Model file for the job. Use its own axes, mm. Face numbers are marked on the shaded views. Give positions to 0.01 mm unless a question says otherwise; leave off trailing zeros. Order: outer loops, then holes, each group sorted by start corner. A loop starts at its lowest first (then second) coordinate and runs counter-clockwise, first axis right, second up. Notation, with made-up numbers: (-24.75, -39) -> (30.25, -39) arc R24 ccw to (30.25, -29) -> close; hole circle Ø2 at (15.5, -36.75). An arc over 180 degrees is marked (long way). Answer in a Markdown table with one row per item. Add a question column.
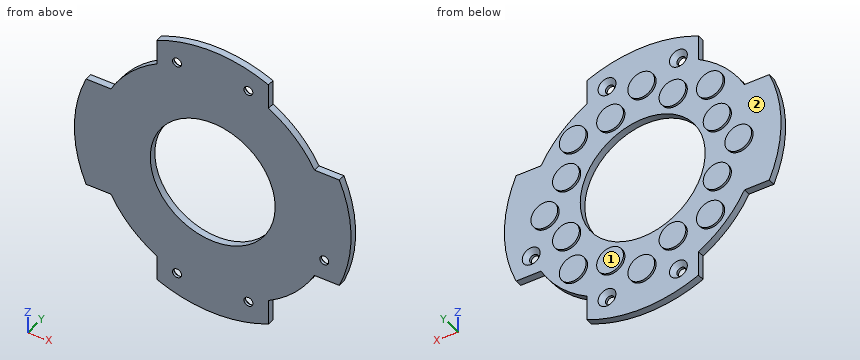
from build123d import *

# Parameters (mm, degrees)
SKETCH1_R           = 7
BOSS_EXTRUDE1_DEPTH = 0.7874
SKETCH2_R           = 1.5
BOSS_EXTRUDE2_DEPTH = 0.25
SKETCH3_R           = 0.5
CUT_EXTRUDE1_DEPTH  = 1.7874
CHAMFER1_SIZE       = 0.5


with BuildPart() as part:
    # Sketch1 → Boss-Extrude1 (new body)
    with BuildSketch(Plane(origin=(0, 0, 0), x_dir=(1, 0, 0), z_dir=(0, 1, 0))):
        with BuildLine():
            Line((-6.25, 14.184057953), (-6.25, 11.399013115))
            ThreePointArc((-6.25, 11.399013115), (-9.192388155, 9.192388155), (-11.399013115, 6.25))
            Line((-11.399013115, 6.25), (-14.184057953, 6.25))
            ThreePointArc((-14.184057953, 6.25), (-15.5, 0), (-14.184057953, -6.25))
            Line((-14.184057953, -6.25), (-11.399013115, -6.25))
            ThreePointArc((-11.399013115, -6.25), (-9.192388155, -9.192388155), (-6.25, -11.399013115))
            Line((-6.25, -11.399013115), (-6.25, -14.184057953))
            ThreePointArc((-6.25, -14.184057953), (0, -15.5), (6.25, -14.184057953))
            Line((6.25, -14.184057953), (6.25, -11.399013115))
            ThreePointArc((6.25, -11.399013115), (9.192388155, -9.192388155), (11.399013115, -6.25))
            Line((11.399013115, -6.25), (14.184057953, -6.25))
            ThreePointArc((14.184057953, -6.25), (15.5, 0), (14.184057953, 6.25))
            Line((14.184057953, 6.25), (11.399013115, 6.25))
            ThreePointArc((11.399013115, 6.25), (9.192388155, 9.192388155), (6.25, 11.399013115))
            Line((6.25, 11.399013115), (6.25, 14.184057953))
            ThreePointArc((6.25, 14.184057953), (0, 15.5), (-6.25, 14.184057953))
        make_face()
        Circle(SKETCH1_R, mode=Mode.SUBTRACT)
    extrude(amount=BOSS_EXTRUDE1_DEPTH)

    # Sketch2 → Boss-Extrude2 (add)
    with BuildSketch(Plane(origin=(0, 0.7874, 0), x_dir=(1, 0, 0), z_dir=(0, 1, 0))):
        with Locations((0, 10.865)):
            Circle(SKETCH2_R)
        with Locations((-3.495813155, 8.439639529)):
            Circle(SKETCH2_R)
        with Locations((-10.865, 0)):
            Circle(SKETCH2_R)
        with Locations((-8.439639529, 3.495813155)):
            Circle(SKETCH2_R)
        with Locations((-7.682715178, 7.682715178)):
            Circle(SKETCH2_R)
        with Locations((0, -10.865)):
            Circle(SKETCH2_R)
        with Locations((-3.495813155, -8.439639529)):
            Circle(SKETCH2_R)
        with Locations((-7.682715178, -7.682715178)):
            Circle(SKETCH2_R)
        with Locations((-8.439639529, -3.495813155)):
            Circle(SKETCH2_R)
        with Locations((3.495813155, 8.439639529)):
            Circle(SKETCH2_R)
        with Locations((7.682715178, 7.682715178)):
            Circle(SKETCH2_R)
        with Locations((8.439639529, 3.495813155)):
            Circle(SKETCH2_R)
        with Locations((10.865, 0)):
            Circle(SKETCH2_R)
        with Locations((8.439639529, -3.495813155)):
            Circle(SKETCH2_R)
        with Locations((7.682715178, -7.682715178)):
            Circle(SKETCH2_R)
        with Locations((3.495813155, -8.439639529)):
            Circle(SKETCH2_R)
    extrude(amount=BOSS_EXTRUDE2_DEPTH)

    # Sketch3 → Cut-Extrude1 (cut, through all)
    with BuildSketch(Plane(origin=(0, 0.7874, 0), x_dir=(1, 0, 0), z_dir=(0, 1, 0))):
        with Locations((-4, 12.5)):
            Circle(SKETCH3_R)
        with Locations((4, 12.5)):
            Circle(SKETCH3_R)
        with Locations((4, -12.5)):
            Circle(SKETCH3_R)
        with Locations((-4, -12.5)):
            Circle(SKETCH3_R)
        with Locations((12.5, 4)):
            Circle(SKETCH3_R)
    extrude(amount=-CUT_EXTRUDE1_DEPTH, mode=Mode.SUBTRACT)

    # Chamfer1
    chamfer1_edges = [part.edges().sort_by_distance(p)[0] for p in [
        (-4.5, 0.7874, -12.5),
        (3.5, 0.7874, -12.5),
        (3.5, 0.7874, 12.5),
        (-4.5, 0.7874, 12.5),
        (12, 0.7874, -4),
    ]]
    chamfer(chamfer1_edges, length=CHAMFER1_SIZE)


solid = part.part
Item 1: Two-plate mould, pull along X, no slides. Class the marked faces 1 and 2: pulls with the +X half, pulls with the -X half, needs draft (parallel to the pull), parting line crosses it, or undercut.
Item 2: Saw through at B-B on x = 0. List the corners of the cut face in (y, z) (3 decimals), plus the area to 3 significant figures.
Item 3: Saw through at A-A on z = 0. List the corners of the cut face in (x, y) (3 decimals), plus the area to 3 significant figures.
Item 4: Saw through at D-D on z = -4. List the corners of the cut face in (x, y).
Item 5: Wall check: line 1 (X direction, y = 0.1, z = -12.5); line 2 (Z direction, x = 4, y = 0.25); line 3 (X direction, y = 0.25, z = -4). Give the ranges that are in metal, low to high.
Item 6: Saw through at C-C on x = -4. List the corners of the cut face in (y, z).
Item 7: Pin check, flat tips, straight feed: pin 1 Ø0.6 at (y, z) = (0.5, 12) entering from -X; pin 2 Ø0.6 at (x, y) = (12.5, 0.5) entering from +Z; pin 3 Ø0.6 at (y, z) = (0.5, -13.5) entering from +X; pin 4 Ø8.5 at (x, z) = (0, 0) entering from -Y. Stop position of each tip, or through.
Evaluation:
| question | item | result |
|---|---|---|
| 1 | face 1 | needs draft |
| 1 | face 2 | undercut |
| 2 | outline | (0, -15.5) -> (0.787, -15.5) -> (0.787, -12.365) -> (1.037, -12.365) -> (1.037, -9.365) -> (0.787, -9.365) -> (0.787, -7) -> (0, -7) -> close; (0, 7) -> (0.787, 7) -> (0.787, 9.365) -> (1.037, 9.365) -> (1.037, 12.365) -> (0.787, 12.365) -> (0.787, 15.5) -> (0, 15.5) -> close |
| 2 | area | 14.9 mm2 |
| 3 | outline | (-15.5, 0) -> (-7, 0) -> (-7, 0.787) -> (-9.365, 0.787) -> (-9.365, 1.037) -> (-12.365, 1.037) -> (-12.365, 0.787) -> (-15.5, 0.787) -> close; (7, 0) -> (15.5, 0) -> (15.5, 0.787) -> (12.365, 0.787) -> (12.365, 1.037) -> (9.365, 1.037) -> (9.365, 0.787) -> (7, 0.787) -> close |
| 3 | area | 14.9 mm2 |
| 4 | outline | (-14.97, 0) -> (-5.74, 0) -> (-5.74, 0.79) -> (-7.03, 0.79) -> (-7.03, 1.04) -> (-9.85, 1.04) -> (-9.85, 0.79) -> (-14.97, 0.79) -> close; (5.74, 0) -> (12, 0) -> (12, 0.29) -> (11.5, 0.79) -> (9.85, 0.79) -> (9.85, 1.04) -> (7.03, 1.04) -> (7.03, 0.79) -> (5.74, 0.79) -> close; (13, 0) -> (14.97, 0) -> (14.97, 0.79) -> (13.5, 0.79) -> (13, 0.29) -> close |
| 5 | line 1 | x = -6.25 to -4.5, -3.5 to 3.5, 4.5 to 6.25 |
| 5 | line 2 | z = -14.97 to -13, -12 to -5.74, 5.74 to 12, 13 to 14.97 |
| 5 | line 3 | x = -14.97 to -5.74, 5.74 to 12, 13 to 14.97 |
| 6 | outline | (0, -14.97) -> (0.79, -14.97) -> (0.79, -13.5) -> (0.29, -13) -> (0, -13) -> close; (0, -12) -> (0.29, -12) -> (0.79, -11.5) -> (0.79, -9.85) -> (1.04, -9.85) -> (1.04, -7.03) -> (0.79, -7.03) -> (0.79, -5.74) -> (0, -5.74) -> close; (0, 5.74) -> (0.79, 5.74) -> (0.79, 7.03) -> (1.04, 7.03) -> (1.04, 9.85) -> (0.79, 9.85) -> (0.79, 11.5) -> (0.29, 12) -> (0, 12) -> close; (0, 13) -> (0.29, 13) -> (0.79, 13.5) -> (0.79, 14.97) -> (0, 14.97) -> close |
| 7 | pin 1 | stops at x = -6.25 |
| 7 | pin 2 | stops at z = 6.25 |
| 7 | pin 3 | stops at x = 6.25 |
| 7 | pin 4 | passes through |
